```python
from build123d import *

# Parameters (mm, degrees)
SKETCH1_R           = 7.5
BOSS_EXTRUDE2_DEPTH = 80
SKETCH3_R           = 2.5
CUT_EXTRUDE1_DEPTH  = 2000


with BuildPart() as part:
    # Sketch1 → Boss-Extrude2 (new body)
    with BuildSketch(Plane.XY):
        with BuildLine():
            Line((0, 0), (-17.5, 0))
            Line((-17.5, 0), (-17.5, 5))
            ThreePointArc((-17.5, 5), (-27.5, 15), (-37.5, 5))
            Line((-37.5, 5), (-37.5, 0))
            Line((-37.5, 0), (-55, 0))
            Line((-55, 0), (-55, -10))
            Line((-55, -10), (0, -10))
            Line((0, -10), (0, 0))
        make_face()
        with Locations((-27.5, 5)):
            Circle(SKETCH1_R, mode=Mode.SUBTRACT)
    extrude(amount=BOSS_EXTRUDE2_DEPTH)

    # Sketch3 → Cut-Extrude1 (cut)
    with BuildSketch(Plane(origin=(0, 0, 0), x_dir=(1, 0, 0), z_dir=(0, 1, 0))):
        with Locations(Location((-8.75, -10, 0), (0, 0, 270))):
            Circle(SKETCH3_R)
        with Locations(Location((-8.75, -30, 0), (0, 0, 270))):
            Circle(SKETCH3_R)
        with Locations(Location((-8.75, -50, 0), (0, 0, 270))):
            Circle(SKETCH3_R)
        with Locations(Location((-8.75, -70, 0), (0, 0, 270))):
            Circle(SKETCH3_R)
        with Locations(Location((-46.25, -70, 0), (0, 0, 180))):
            Circle(SKETCH3_R)
        with Locations(Location((-46.25, -50, 0), (0, 0, 180))):
            Circle(SKETCH3_R)
        with Locations(Location((-46.25, -30, 0), (0, 0, 180))):
            Circle(SKETCH3_R)
        with Locations(Location((-46.25, -10, 0), (0, 0, 180))):
            Circle(SKETCH3_R)
    extrude(amount=-CUT_EXTRUDE1_DEPTH, mode=Mode.SUBTRACT)


solid = part.part
```
Can you work these out from the model? Positions are in its coordinate system, mm. A direction names the side the tool comes from. Round coordinates to 2 decimals unless told otherwise and drop trailing zeros. Loops run counter-clockwise (first coordinate to the right, second up) from the corner with the lowest first, then second, coordinate; pieces in that order, holes last. Notation, with made-up numbers: (14.25, 43.25) -> (65.25, 43.25) arc R30 ccw to (65.25, 67.25) -> close; hole circle Ø5 at (9, 74). An arc over 180 degrees is marked (long way). One line per item, written item: value. Start each with the question number.
1. If we section it at C-C, the plane y = -8: Give the number of separate pieces and of enclosed holes in the cut face, then the cut area to 3 significant figures.
2. For pin 1 (8 mm diameter, centred on x = -46.25, z = 10, fed in from +Y); pin 2 (4.5 mm diameter, centred on x = -46.25, z = 30, fed in from -Y); pin 3 (2 mm diameter, centred on y = 4, z = 54, fed in from +X); pin 4 (4 mm diameter, centred on x = -20.5, z = 46.5, fed in from +Y), each with a flat end and sliding along its axis, tell me the tip position at first contact or that it passes through.
3. If I drill on probe 1 along Z at (x, y) = (-46.25, -7); probe 2 along X at (y, z) = (5.5, 39); probe 3 along Z at (x, y) = (-8, -0.75), over which ranges is the centre line in solid material (lowest first)?
4. If we mould it in two halves opening along Z, with no side actions, what happens to faces 1 (the cylindrical face through (-48.56, -4.93, 49.04)), 2 (the flat face through (-37.5, 3, 39)), 3 (the flat face through (-28, -3, 80))? For each: pulls with the +Z half, pulls with the -Z half, needs draft (parallel to the pull), parting line crosses it, or undercut.
5. If we section it at D-D, the plane z = 24: Write out the boundary of the cut face in (x, y).
6. For faces 4 (the flat face through (-17.5, 2, 39)), 5 (the flat face through (-46, 0, 39)), 6 (the cylindrical face through (-48.56, -4.93, 9.04)), which set-ups out of +Z, -Z, +X, -X, +Y, -Y let a thin tool reach every point of the face, with its end or its side?
7. If we section it at A-A, the plane z = 8.5: Write out the boundary of the cut face in (x, y).
8. If we section it at B-B, the plane x = -27.5: Write out the boundary of the cut face in (y, z).
Calculated:
1. separate pieces: 1
1. enclosed holes: 8
1. area: 4,240 mm²
2. pin 1: stops at y = 0
2. pin 2: passes through
2. pin 3: stops at x = -17.5
2. pin 4: stops at y = 13.66
3. probe 1: z = 0 to 7.5, 12.5 to 27.5, 32.5 to 47.5, 52.5 to 67.5, 72.5 to 80
3. probe 2: x = -37.49 to -34.98, -20.02 to -17.51
3. probe 3: z = 0 to 7.62, 12.38 to 27.62, 32.38 to 47.62, 52.38 to 67.62, 72.38 to 80
4. face 1: undercut
4. face 2: needs draft
4. face 3: pulls with the +Z half
5. outline: (-55, -10) -> (0, -10) -> (0, 0) -> (-17.5, 0) -> (-17.5, 5) arc R10 ccw to (-37.5, 5) -> (-37.5, 0) -> (-55, 0) -> close; hole circle Ø15 at (-27.5, 5)
6. face 4: +Z, -Z, +X, +Y
6. face 5: +Z, -Z, -X, +Y
6. face 6: +Y, -Y
7. outline: (-55, -10) -> (-48.25, -10) -> (-48.25, 0) -> (-55, 0) -> close; (-44.25, -10) -> (-10.75, -10) -> (-10.75, 0) -> (-17.5, 0) -> (-17.5, 5) arc R10 ccw to (-37.5, 5) -> (-37.5, 0) -> (-44.25, 0) -> close; (-6.75, -10) -> (0, -10) -> (0, 0) -> (-6.75, 0) -> close; hole circle Ø15 at (-27.5, 5)
8. outline: (-10, 0) -> (-2.5, 0) -> (-2.5, 80) -> (-10, 80) -> close; (12.5, 0) -> (15, 0) -> (15, 80) -> (12.5, 80) -> close
